```python
from build123d import *

# Parameters (mm, degrees)
SKETCH1_R           = 2.5
SKETCH1_R_2         = 1
SKETCH1_R_3         = 1.5
SKETCH1_W           = 22.5
SKETCH1_H           = 11.8
BOSS_EXTRUDE1_DEPTH = 8.3
FILLET1_R           = 2


with BuildPart() as part:
    # Sketch1 → Boss-Extrude1 (new body)
    with BuildSketch(Plane(origin=(0, 0, 0), x_dir=(1, 0, 0), z_dir=(0, 1, 0))):
        with BuildLine():
            Line((-15, 20), (-13, 20))
            Line((-13, 20), (-11, 34))
            Line((-11, 34), (11, 34))
            Line((11, 34), (13, 20))
            Line((13, 20), (15, 20))
            ThreePointArc((15, 20), (22.071067812, 17.071067812), (25, 10))
            Line((25, 10), (25, -10))
            ThreePointArc((25, -10), (22.071067812, -17.071067812), (15, -20))
            Line((15, -20), (-15, -20))
            ThreePointArc((-15, -20), (-22.071067812, -17.071067812), (-25, -10))
            Line((-25, -10), (-25, 10))
            ThreePointArc((-25, 10), (-22.071067812, 17.071067812), (-15, 20))
        make_face()
        with Locations(Location((-12.5, 10, 0), (0, 0, 90))):
            Circle(SKETCH1_R, mode=Mode.SUBTRACT)
        with Locations(Location((12.5, 10, 0), (0, 0, 90))):
            Circle(SKETCH1_R, mode=Mode.SUBTRACT)
        with Locations(Location((13.65, -10, 0), (0, 0, 90))):
            Circle(SKETCH1_R_2, mode=Mode.SUBTRACT)
        with Locations(Location((-13.65, -10, 0), (0, 0, 90))):
            Circle(SKETCH1_R_2, mode=Mode.SUBTRACT)
        with Locations(Location((8, 30, 0), (0, 0, 90))):
            Circle(SKETCH1_R_3, mode=Mode.SUBTRACT)
        with Locations(Location((-8, 30, 0), (0, 0, 90))):
            Circle(SKETCH1_R_3, mode=Mode.SUBTRACT)
        with Locations((0, -10)):
            Rectangle(SKETCH1_W, SKETCH1_H, mode=Mode.SUBTRACT)
    extrude(amount=BOSS_EXTRUDE1_DEPTH)

    # Fillet1
    fillet1_edges = [part.edges().sort_by_distance(p)[0] for p in [
        (-13, 4.15, -20),
        (-11, 4.15, -34),
        (11, 4.15, -34),
        (13, 4.15, -20),
    ]]
    fillet(fillet1_edges, radius=FILLET1_R)


solid = part.part
```
Geometry check sheet. Reference: the model listing, model coordinates, mm. A direction names the side the tool comes from. Give positions to 0.01 mm unless a question says otherwise; leave off trailing zeros. Order: outer loops, then holes, each group sorted by start corner. A loop starts at its lowest first (then second) coordinate and runs counter-clockwise, first axis right, second up. Notation, with made-up numbers: (1.5, 25) - (34.5, 25) arc R18 ccw to (34.5, 45) - close; hole circle Ø6 at (-22, 81.5). An arc over 180 degrees is marked (long way). Write item = value, one per line. Start each with the question number.
1) Access from +Z, -Z, +X, -X, +Y, -Y to the whole of each face (thin tool, end or side, straight path). Record for faces 4 (the cylindrical face through (-22.15, 4.09, -16.99)), 5 (the flat face through (0, 4, 15.9)).
2) Section check A-A (x = 0.5). Enter the section's corners in (y, z).
3) Section check D-D (x = -8). Enter the section's corners in (y, z), then the cut area to 3 significant figures.
4) Gauge pin test, flat ends, axial feed: pin 1 Ø1.6 at (x, z) = (13.65, 10) entering from +Y; pin 2 Ø5 at (x, z) = (-20, 12) entering from -Y; pin 3 Ø3 at (y, z) = (2, -14.5) entering from -X. Record the tip position at first contact, or that the pin passes through.
5) Section check B-B (z = 5). Enter the section's corners in (x, y).
6) Draft check along X on faces 1 (the flat face through (0, 4, 4.1)), 2 (the flat face through (0, 0, -7)), 3 (the cylindrical face through (21.99, 4.09, -17.15)). Enter one of: released by +X, released by -X, zero draft, split by the parting line, or undercut.
7) Scan lines: L1, parallel to X at y = 5.25, z = 10; L2, parallel to X at y = 3, z = -10; L3, parallel to Z at x = -5.5, y = 5.5. Record each from-to range of solid material in increasing order.
8) Section check C-C (y = 1.5). Enter the section's corners in (x, z), then the cut area to 3 significant figures.
Geometry check:
q1.face_4 = -Z, -X, +Y, -Y
q1.face_5 = +Y, -Y
q2.outline = (0, -34) - (8.3, -34) - (8.3, 4.1) - (0, 4.1) - close; (0, 15.9) - (8.3, 15.9) - (8.3, 20) - (0, 20) - close
q3.outline = (0, -34) - (8.3, -34) - (8.3, -31.5) - (0, -31.5) - close; (0, -28.5) - (8.3, -28.5) - (8.3, 4.1) - (0, 4.1) - close; (0, 15.9) - (8.3, 15.9) - (8.3, 20) - (0, 20) - close
q3.area = 325 mm2
q4.pin_1 = through
q4.pin_2 = 0
q4.pin_3 = -24.54
q5.outline = (-25, 0) - (-11.25, 0) - (-11.25, 8.3) - (-25, 8.3) - close; (11.25, 0) - (25, 0) - (25, 8.3) - (11.25, 8.3) - close
q6.face_1 = undercut
q6.face_2 = zero draft
q6.face_3 = released by +X
q7.L1 = -25 to -14.65, -12.65 to -11.25, 11.25 to 12.65, 14.65 to 25
q7.L2 = -25 to -15, -10 to 10, 15 to 25
q7.L3 = -34 to 4.1, 15.9 to 20
q8.outline = (-25, -10) arc R10 ccw to (-15, -20) - (-14.73, -20) arc R2 cw to (-12.75, -21.72) - (-11.25, -32.28) arc R2 ccw to (-9.27, -34) - (9.27, -34) arc R2 ccw to (11.25, -32.28) - (12.75, -21.72) arc R2 cw to (14.73, -20) - (15, -20) arc R10 ccw to (25, -10) - (25, 10) arc R10 ccw to (15, 20) - (-15, 20) arc R10 ccw to (-25, 10) - close; hole circle Ø5 at (-12.5, -10); hole circle Ø2 at (-13.65, 10); hole (-11.25, 4.1) - (11.25, 4.1) - (11.25, 15.9) - (-11.25, 15.9) - close; hole circle Ø3 at (-8, -30); hole circle Ø3 at (8, -30); hole circle Ø5 at (12.5, -10); hole circle Ø2 at (13.65, 10)
q8.area = 1,920 mm2
